Input: part model. Units: mm. Frame: model coordinates. Give positions to 0.01 mm unless a question says otherwise; leave off trailing zeros. Write each loop counter-clockwise with the first axis right and the second up, starting at its lowest first coordinate (ties: lowest second). Pieces come first, ordered by that corner, then holes. Notation, with made-up numbers: (2, 14) -> (43, 14) arc R11 cw to (43, 34) -> close; hole circle Ø8 at (85, 22.5). An arc over 180 degrees is marked (long way). Return JSON: item names as keys, results as strings. Group by question number.
Item 1: Section A-A, the plane y = 0. Return loops of the section in (x, z).
Item 2: Section C-C, the plane y = 50. Return loops of the section in (x, z), then the cut area to 3 significant figures.
Item 3: Section D-D, the plane x = 1.75. Count the separate pieces of the cut face and the enclosed holes in it, then the cut area to 3 significant figures.
Item 4: Line query: line 1 (Y direction, x = 1.45, z = 36); line 2 (Z direction, x = 1.15, y = -3.5); line 3 (Y direction, x = 2.3, z = 28). Output: solid intervals per line, ascending. Write a range as [from, to].
Item 5: Mould query, pull axis Z, two halves, no side actions, for faces 1 (the face through (4, 1, 1)), 2 (the face through (1.97, -46.42, 60.54)), 3 (the face through (1.972, -11.944, 10.311)). Classes: released by +Z, released by -Z, zero draft, split by the parting line, or undercut.
Item 6: Pin query (flat end, axial travel): P1, Ø1.5, axis at x = 3.5, y = -57.5, coming from the +Z side; P2, Ø4, axis at y = -13.5, z = -9.5, coming from the -X side; P3, Ø1.5, axis at x = 3, z = 46.5, coming from the +Y side. Return the tip coordinate at first contact, or that it passes through.
Item 7: Section B-B, the plane z = -23. Return loops of the section in (x, y).
from build123d import *

# Parameters (mm, degrees)
SKETCH1_R           = 76.29
SKETCH1_R_2         = 4
SKETCH1_R_3         = 14.75
SKETCH1_R_4         = 1.75
BOSS_EXTRUDE1_DEPTH = 4


with BuildPart() as part:
    # Sketch1 → Boss-Extrude1 (new body)
    with BuildSketch(Plane(origin=(0, 0, 0), x_dir=(0, 0, -1), z_dir=(1, 0, 0))):
        Circle(SKETCH1_R)
        with Locations((0, 50)):
            Circle(SKETCH1_R_2, mode=Mode.SUBTRACT)
        with Locations((43.301270189, -25)):
            Circle(SKETCH1_R_2, mode=Mode.SUBTRACT)
        with Locations((-43.301270189, -25)):
            Circle(SKETCH1_R_2, mode=Mode.SUBTRACT)
        with Locations((23, 0)):
            Circle(SKETCH1_R_3, mode=Mode.SUBTRACT)
        with Locations(Location((-23, 0, 0), (0, 0, 180))):
            Circle(SKETCH1_R_3, mode=Mode.SUBTRACT)
        with Locations((36.496900686, 13.496900686)):
            Circle(SKETCH1_R_4, mode=Mode.SUBTRACT)
        with Locations((36.496900686, -13.496900686)):
            Circle(SKETCH1_R_4, mode=Mode.SUBTRACT)
        with Locations((9.503099314, -13.496900686)):
            Circle(SKETCH1_R_4, mode=Mode.SUBTRACT)
        with Locations((9.503099314, 13.496900686)):
            Circle(SKETCH1_R_4, mode=Mode.SUBTRACT)
        with Locations(Location((-36.496900686, -13.496900686, 0), (0, 0, 180))):
            Circle(SKETCH1_R_4, mode=Mode.SUBTRACT)
        with Locations(Location((-9.503099314, -13.496900686, 0), (0, 0, 180))):
            Circle(SKETCH1_R_4, mode=Mode.SUBTRACT)
        with Locations(Location((-9.503099314, 13.496900686, 0), (0, 0, 180))):
            Circle(SKETCH1_R_4, mode=Mode.SUBTRACT)
        with Locations(Location((-36.496900686, 13.496900686, 0), (0, 0, 180))):
            Circle(SKETCH1_R_4, mode=Mode.SUBTRACT)
    extrude(amount=BOSS_EXTRUDE1_DEPTH)


solid = part.part
Answer below:
{
 "1": {"outline": "(0, -76.29) -> (4, -76.29) -> (4, -37.75) -> (0, -37.75) -> close; (0, -8.25) -> (4, -8.25) -> (4, 8.25) -> (0, 8.25) -> close; (0, 37.75) -> (4, 37.75) -> (4, 76.29) -> (0, 76.29) -> close"},
 "2": {"outline": "(0, -57.62) -> (4, -57.62) -> (4, -4) -> (0, -4) -> close; (0, 4) -> (4, 4) -> (4, 57.62) -> (0, 57.62) -> close", "area": "429 mm2"},
 "3": {"separate pieces": "1", "enclosed holes": "13", "area": "16,700 mm2"},
 "4": {"line 1": "y = [-67.26, -15.17], [-11.82, -6.97], [6.97, 11.82], [15.17, 67.26]", "line 2": "z = [-76.21, -37.33], [-8.67, 8.67], [37.33, 76.21]", "line 3": "y = [-70.97, -13.88], [13.88, 70.97]"},
 "5": {"face 1": "zero draft", "face 2": "split by the parting line", "face 3": "undercut"},
 "6": {"P1": "stops at z = 50.99", "P2": "stops at x = 0", "P3": "stops at y = 61.05"},
 "7": {"outline": "(0, -72.74) -> (4, -72.74) -> (4, -14.75) -> (0, -14.75) -> close; (0, 14.75) -> (4, 14.75) -> (4, 72.74) -> (0, 72.74) -> close"}
}
